```python
from build123d import *

# Parameters (mm, degrees)
F0_R     = 2.15
F0_R_2   = 0.95
F1_DEPTH = 4
F3_DEPTH = 25
F4_R     = 1.95
F4_R_2   = 0.95
F5_DEPTH = 4


with BuildPart() as f1:
    # F0 (on Front) → F1 (new body)
    with BuildSketch(Plane.XZ):
        with BuildLine():
            Line((-1.9386593306, 9.96), (-2.9825528163, 0.3230769231))
            ThreePointArc((-2.9825528163, 0.3230769231), (0, -3), (2.9825528163, 0.3230769231))
            Line((2.9825528163, 0.3230769231), (1.9386593306, 9.96))
            ThreePointArc((1.9386593306, 9.96), (0, 11.7), (-1.9386593306, 9.96))
        make_face()
        Circle(F0_R, mode=Mode.SUBTRACT)
        with Locations((0, 9.75)):
            Circle(F0_R_2, mode=Mode.SUBTRACT)
    extrude(amount=F1_DEPTH)

    # F2 (on face) → F3 (cut)
    with BuildSketch(Plane.XZ.offset(4)):
        with BuildLine():
            ThreePointArc((1.3896030661, 8.5287288103), (0, 7.9), (-1.3896030661, 8.5287288103))
            Line((-1.3896030661, 8.5287288103), (-2.0548350523, 2.3874993))
            ThreePointArc((-2.0548350523, 2.3874993), (0, 3.15), (2.0548350523, 2.3874993))
            Line((2.0548350523, 2.3874993), (1.3896030661, 8.5287288103))
        make_face()
    extrude(amount=-F3_DEPTH, mode=Mode.SUBTRACT)

    # F4 (on face) → F5 (join)
    with BuildSketch(Plane.XZ.offset(4)):
        with Locations((0, 9.75)):
            Circle(F4_R)
        with Locations((0, 9.75)):
            Circle(F4_R_2, mode=Mode.SUBTRACT)
    extrude(amount=F5_DEPTH)


solid = f1.part
```
Can you work these out from the model? Positions are in its coordinate system, mm. Coordinates: 2 decimals unless noted, no trailing zeros. Loops run counter-clockwise (first coordinate to the right, second up) from the corner with the lowest first, then second, coordinate; pieces in that order, holes last. Notation, with made-up numbers: (4, 13.25) -> (10, 13.25) arc R18 cw to (10, 46.25) -> close; hole circle Ø7 at (63, 71.5). An arc over 180 degrees is marked (long way). Put each result on its own line as item: value. Start each with the question number.
Q1. Thinking about a two-plate mould opening in Z: for faces 1 (the face through (0, -2, 7.9)), 2 (the face through (0, 0, 2.8)), 3 (the face through (-2.453, -1.972, 5.209)), which applies, pulls with the +Z half, pulls with the -Z half, needs draft (parallel to the pull), parting line crosses it, or undercut?
Q2. I want a section at A-A (x = 0). Write out the boundary of the cut face in (y, z), plus the area to 3 significant figures.
Q3. If I drill on line 1 (Z direction, x = -1, y = -2.25); line 2 (Z direction, x = 0, y = -6); line 3 (Z direction, x = 0.75, y = -3.25), over which ranges is the centre line in solid material (lowest first)? Write a range as [from, to].
Q4. I want a section at C-C (y = -1). Write out the boundary of the cut face in (x, z), plus the area to 3 significant figures.
Q5. I'm going to push flat-ended pins straight in: P1, Ø1, axis at y = -3, z = 3.5, coming from the -X side; P2, Ø1, axis at x = 0, z = -1, coming from the +Y side; P3, Ø1.8, axis at x = 1.5, z = 1.5, coming from the -Y side. Where does each tip first touch, or does it pass through?
Q6. I want a section at B-B (z = 0). Write out the boundary of the cut face in (x, y), plus the area to 3 significant figures.
Q7. I want a section at D-D (y = -7.5). Write out the boundary of the cut face in (x, z).
Taken from the geometry:
1. face 1: undercut
1. face 2: needs draft
1. face 3: pulls with the +Z half
2. outline: (-8, 7.8) -> (-4, 7.8) -> (-4, 7.9) -> (0, 7.9) -> (0, 8.8) -> (-8, 8.8) -> close; (-8, 10.7) -> (0, 10.7) -> (0, 11.7) -> (-8, 11.7) -> close; (-4, -3) -> (0, -3) -> (0, -2.15) -> (-4, -2.15) -> close; (-4, 2.15) -> (0, 2.15) -> (0, 3.15) -> (-4, 3.15) -> close
2. area: 23.0 mm2
3. line 1: z = [-2.83, -1.9], [1.9, 2.99], [8.19, 11.42]
3. line 2: z = [7.8, 8.8], [10.7, 11.7]
3. line 3: z = [-2.9, -2.01], [2.01, 3.06], [8.06, 9.17], [10.33, 11.55]
4. outline: (-2.98, 0.32) arc R3 ccw (long way) to (2.98, 0.32) -> (1.94, 9.96) arc R1.95 ccw to (-1.94, 9.96) -> close; hole circle Ø4.3 at (0, 0); hole (-2.05, 2.39) arc R3.15 cw to (2.05, 2.39) -> (1.39, 8.53) arc R1.85 cw to (-1.39, 8.53) -> close; hole circle Ø1.9 at (0, 9.75)
4. area: 33.5 mm2
5. P1: stops at x = -2.69
5. P2: passes through
5. P3: stops at y = -4
6. outline: (-3, -4) -> (-2.15, -4) -> (-2.15, 0) -> (-3, 0) -> close; (2.15, -4) -> (3, -4) -> (3, 0) -> (2.15, 0) -> close
6. area: 6.80 mm2
7. outline: circle Ø3.9 at (0, 9.75); hole circle Ø1.9 at (0, 9.75)
